Source: three-view drawing plus pictorial views. Frame: mm from the lowest corner of the part. A direction names the side the tool comes from. Coordinates: 2 decimals unless noted, no trailing zeros. Loops run counter-clockwise (first coordinate to the right, second up) from the corner with the lowest first, then second, coordinate; pieces in that order, holes last. Notation, with made-up numbers: (42.5, 75.5) - (58.5, 75.5) arc R23 cw to (58.5, 91.5) - close; hole circle Ø9 at (-34, 48). An arc over 180 degrees is marked (long way). Return JSON: item names as keys, results as strings.
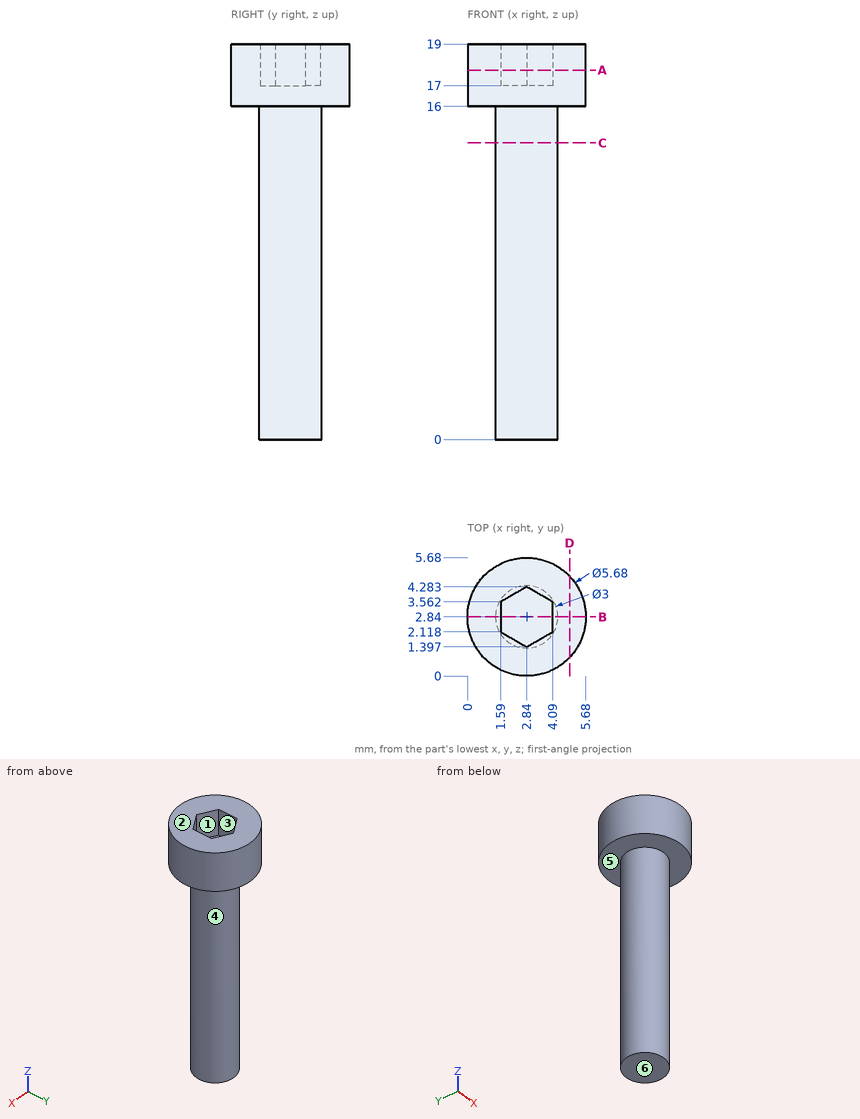
Item 1: Mould query, pull axis Y, two halves, no side actions, for the marked faces 1, 2, 3 and 4. Classes: +Y half, -Y half, draft (parallel to the pull), parting line (faces both ways), or undercut.
Worked out:
{"face 1": "undercut", "face 2": "draft", "face 3": "undercut", "face 4": "parting line"}
Item 2: First-contact query: pin 1 Ø1 at (x, y) = (3, 3) entering from +Z; pin 2 Ø1 at (x, z) = (4, 9.5) entering from +Y; pin 3 Ø3 at (y, z) = (4, 10) entering from -X. Flat tips, straight axial feed; report the tip coordinate or a pass-through.
Worked out:
{"pin 1": "z = 17", "pin 2": "y = 4.19", "pin 3": "x = 1.34"}
Item 3: Ray query, probe 1 along Z at (x, y) = (3.7, 4.5); probe 2 along Y at (x, z) = (2.9, 7.5); probe 3 along Y at (x, z) = (2.5, 18). Return the intervals inside material, ascending. Write a range as from..to.
Worked out:
{"probe 1": "16..19", "probe 2": "1.34..4.34", "probe 3": "0.02..1.59, 4.09..5.66"}
Item 4: Section query A-A, the plane z = 17.75. Return loops of the section in (x, y).
Worked out:
{"outline": "circle Ø5.68 at (2.84, 2.84); hole (1.59, 2.12) - (2.84, 1.4) - (4.09, 2.12) - (4.09, 3.56) - (2.84, 4.28) - (1.59, 3.56) - close"}
Item 5: Reachability of the marked faces 5 and 6 from +Z, -Z, +X, -X, +Y, -Y: full face, straight path, thin tool, end or side. Return the list, or none.
Worked out:
{"face 5": "-Z", "face 6": "-Z, +X, -X, +Y, -Y"}
Item 6: Section query D-D, the plane x = 4.9. Return loops of the section in (y, z) (1 decimal).
Worked out:
{"outline": "(0.9, 16) - (4.8, 16) - (4.8, 19) - (0.9, 19) - close"}
Item 7: Section query C-C, the plane z = 14.25. Return loops of the section in (x, y).
Worked out:
{"outline": "circle Ø3 at (2.84, 2.84)"}
Item 8: Section query B-B, the plane y = 2.84. Return loops of the section in (x, z).
Worked out:
{"outline": "(0, 16) - (1.34, 16) - (1.34, 0) - (4.34, 0) - (4.34, 16) - (5.68, 16) - (5.68, 19) - (4.09, 19) - (4.09, 17) - (1.59, 17) - (1.59, 19) - (0, 19) - close"}
